Print and shaded views of the part. All mm, measured from the part's lowest x, y and z. A direction names the side the tool comes from. Give positions to 0.01 mm unless a question says otherwise; leave off trailing zeros. Loops run counter-clockwise (first coordinate to the right, second up) from the corner with the lowest first, then second, coordinate; pieces in that order, holes last. Notation, with made-up numbers: M -23,47 L 15,47 A8 cw 15,61 Z; hole C 78.5,79 d5. An arc over 180 degrees is marked long. Answer as CSV lines item,"result".
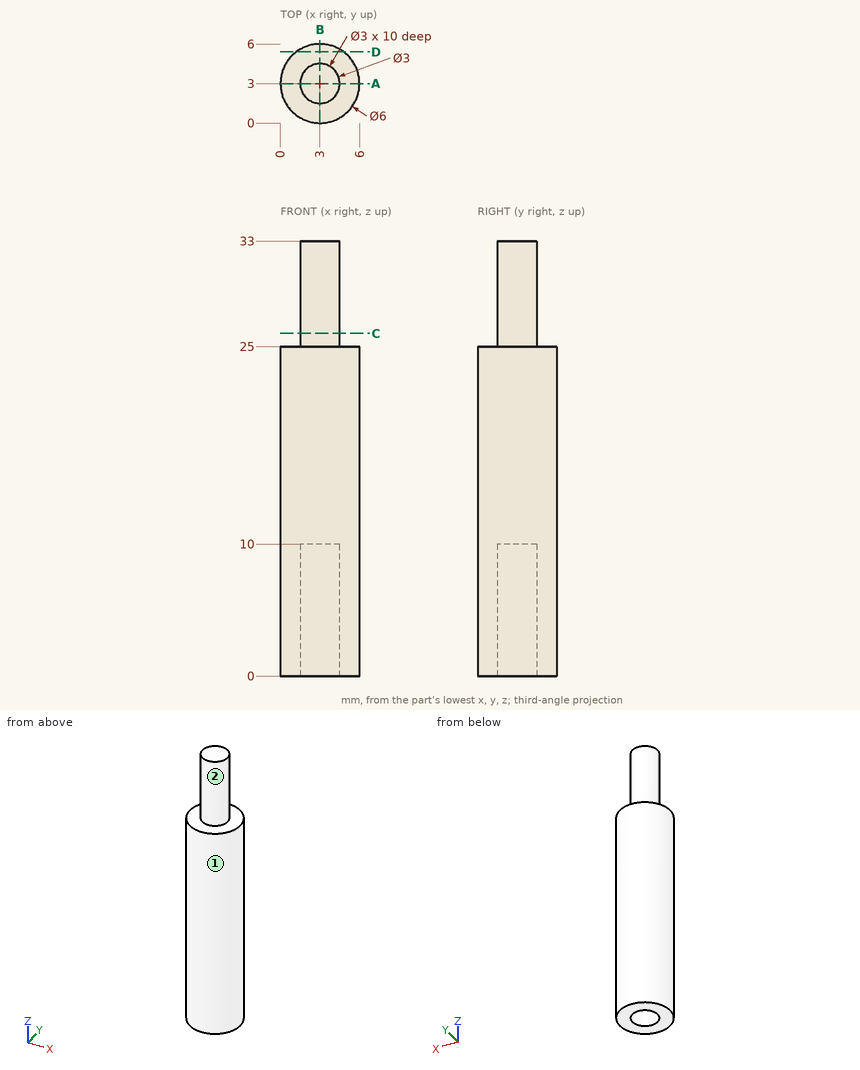
Q1. Cut at D-D (y = 5.4). Write the cut outline in (x, z), and give its area (3 significant figures).
Solution:
outline,"M 1.2,0 L 4.8,0 L 4.8,25 L 1.2,25 Z"
area,"90.0 mm²"
Q2. Cut at A-A (y = 3). Write the cut outline in (x, z).
Solution:
outline,"M 0,0 L 1.5,0 L 1.5,10 L 4.5,10 L 4.5,0 L 6,0 L 6,25 L 4.5,25 L 4.5,33 L 1.5,33 L 1.5,25 L 0,25 Z"
Q3. Cut at C-C (z = 26). Write the cut outline in (x, y), and give its area (3 significant figures).
Solution:
outline,"C 3,3 d3"
area,"7.07 mm²"
Q4. Which spindle directions (+Z, -Z, +X, -X, +Y, -Y) get a long thin tool onto all of the face, cutting with end or side? Do the marked faces 1 and 2. Say none if no direction does.
Solution:
face 1,"+Z, -Z"
face 2,"+Z"
Q5. Wall check: line 1 (Y direction, x = 3, z = 2.5); line 2 (Z direction, x = 1, y = 0.9); line 3 (X direction, y = 3.2, z = 8). Give the ranges that are in metal, low to high. Write a range as [from, to].
Solution:
line 1,"y = [0, 1.5], [4.5, 6]"
line 2,"z = [0, 25]"
line 3,"x = [0.01, 1.51], [4.49, 5.99]"
Q6. Pin check, flat tips, straight feed: P1, Ø2, axis at x = 1, z = 24, coming from the +Y side; P2, Ø2, axis at y = 4.5, z = 19, coming from the +X side; P3, Ø3, axis at y = 2, z = 3.5, coming from the -X side; P4, Ø1.5, axis at x = 2.5, y = 3, coming from the -Z side. Stop position of each tip, or through.
Solution:
P1,"stops at y = 5.83"
P2,"stops at x = 5.96"
P3,"stops at x = 0"
P4,"stops at z = 10"
